from build123d import *

# Parameters (mm, degrees)
F0_W     = 7
F0_H     = 7
F1_DEPTH = 4.5
F3_R     = 1.25
F4_DEPTH = 25
F3_R_2   = 3.25
F5_DEPTH = 4.32


with BuildPart() as f1:
    # F0 (on Top) → F1 (new body)
    with BuildSketch(Plane.XY):
        with Locations((-13.872448, -2.127344)):
            Rectangle(F0_W, F0_H)
    extrude(amount=F1_DEPTH)

    # F3 (on face) → F4 (cut)
    with BuildSketch(Plane(origin=(0, 0, 0), x_dir=(1, 0, 0), z_dir=(0, 0, -1))):
        with Locations((-13.92932, 2.101687)):
            Circle(F3_R)
    extrude(amount=-F4_DEPTH, mode=Mode.SUBTRACT)

    # F3 (on face) → F5 (cut)
    with BuildSketch(Plane(origin=(0, 0, 0), x_dir=(1, 0, 0), z_dir=(0, 0, -1))):
        with Locations((-13.92932, 2.101687)):
            Circle(F3_R_2)
        with Locations((-13.92932, 2.101687)):
            Circle(F3_R, mode=Mode.SUBTRACT)
    extrude(amount=-F5_DEPTH, mode=Mode.SUBTRACT)


solid = f1.part
Geometry check sheet. Reference: the model listing, model coordinates, mm. Round coordinates to 2 decimals unless told otherwise and drop trailing zeros. Write each loop counter-clockwise with the first axis right and the second up, starting at its lowest first coordinate (ties: lowest second). Pieces come first, ordered by that corner, then holes.
Item 1: Mould release check, pull along X, two halves, no side actions. Record for faces 1 (the face through (-14, -5.627, 2)), 2 (the face through (-17.372, -2, 2)), 3 (the face through (-10.83, -3.08, 2.13)), 4 (the face through (-12.5, -2.1, 4.32)): +X half, -X half, draft (parallel to the pull), parting line (faces both ways), or undercut.
Determined:
face 1: draft
face 2: -X half
face 3: undercut
face 4: undercut
Item 2: Section check D-D (x = -12). Record the boundary of the cut face in (y, z), plus the area to 3 significant figures.
Determined:
outline: (-5.63, 0) - (-4.72, 0) - (-4.72, 4.32) - (0.51, 4.32) - (0.51, 0) - (1.37, 0) - (1.37, 4.5) - (-5.63, 4.5) - close
area: 8.90 mm2
Item 3: Section check A-A (y = -2.5). Record the boundary of the cut face in (x, z).
Determined:
outline: (-17.37, 0) - (-17.15, 0) - (-17.15, 4.32) - (-15.11, 4.32) - (-15.11, 4.5) - (-17.37, 4.5) - close; (-12.74, 4.32) - (-10.7, 4.32) - (-10.7, 0) - (-10.37, 0) - (-10.37, 4.5) - (-12.74, 4.5) - close
Item 4: Material ranges on line 1 along Z through (x, y) = (-14.25, -3.75); line 2 along Y through (x, z) = (-11.5, 4.1); line 3 along X through (y, z) = (-2.5, 1.75), recorded low to high.
Determined:
line 1: z = 4.32 to 4.5
line 2: y = -5.63 to -4.26, 0.06 to 1.37
line 3: x = -17.37 to -17.15, -10.7 to -10.37
Item 5: Section check C-C (z = 3.7). Record the boundary of the cut face in (x, y), plus the area to 3 significant figures.
Determined:
outline: (-17.37, -5.63) - (-10.37, -5.63) - (-10.37, 1.37) - (-17.37, 1.37) - close; hole circle Ø6.5 at (-13.93, -2.1)
area: 15.8 mm2
Item 6: Section check B-B (x = -14). Record the boundary of the cut face in (y, z).
Determined:
outline: (-5.63, 0) - (-5.35, 0) - (-5.35, 4.32) - (-3.35, 4.32) - (-3.35, 4.5) - (-5.63, 4.5) - close; (-0.85, 4.32) - (1.15, 4.32) - (1.15, 0) - (1.37, 0) - (1.37, 4.5) - (-0.85, 4.5) - close
